```python
from build123d import *

# Parameters (mm, degrees)
CUT_EXTRUDE1_DEPTH      = 7
CUT_EXTRUDE3_DEPTH      = 7
CUT_EXTRUDE3_DEPTH_BACK = 7
SKETCH9_R               = 0.79375


with BuildPart() as part:
    # Sketch2 → Revolve1 (revolve)
    with BuildSketch(Plane(origin=(0, 0, 0), x_dir=(0, 0, -1), z_dir=(1, 0, 0))):
        Polygon((-12, 0), (-12, 6.1), (-11.6, 6.5), (-4.4, 6.5), (-4, 6.1), (-4, 4), (10.75, 4), (12, 2.75), (12, 0), align=None)
    revolve(axis=Axis((0, 0, -12), (0, 0, 1)))

    # Sketch3 → Cut-Extrude1 (cut)
    with BuildSketch(Plane.XY.offset(12)):
        Polygon((3, -1.732050808), (3, 1.732050808), (0, 3.464101615), (-3, 1.732050808), (-3, -1.732050808), (0, -3.464101615), align=None)
    extrude(amount=-CUT_EXTRUDE1_DEPTH, mode=Mode.SUBTRACT)

    # Cut-Extrude2 cone 1 section (through the dimple's axis) → Cut-Extrude2 (revolve, cut)
    with BuildSketch(Plane(origin=(0, 0, 12), x_dir=(0, -1, 0), z_dir=(1, 0, 0))):
        Polygon((0, 0), (3.464101615, 0), (0, 3.464101615), align=None)
    revolve(axis=Axis((0, 0, 12), (0, 0, -1)), mode=Mode.SUBTRACT)

    # Sketch9 → Cut-Extrude3 (cut, two sides: drawn at the far end of the back side and taken through both)
    with BuildSketch(Plane(origin=(0, 0, 0), x_dir=(1, 0, 0), z_dir=(0, 1, 0)).offset(-CUT_EXTRUDE3_DEPTH_BACK)):
        with Locations(Location((0, -8, 0), (0, 0, 90))):
            Circle(SKETCH9_R)
    extrude(amount=CUT_EXTRUDE3_DEPTH + CUT_EXTRUDE3_DEPTH_BACK, mode=Mode.SUBTRACT)


solid = part.part
```
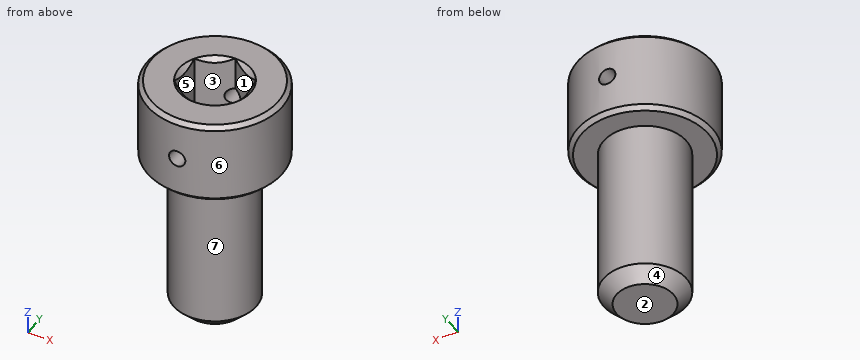
The listing builds one solid part. Answer for the finished solid, in the listing's coordinates (mm). Face numbers are marked on the shaded views. A direction names the side the tool comes from. Coordinates: 2 decimals unless noted, no trailing zeros. Loops run counter-clockwise (first coordinate to the right, second up) from the corner with the lowest first, then second, coordinate; pieces in that order, holes last. Notation, with made-up numbers: (33.5, 14.5) - (79.5, 14.5) arc R16 ccw to (79.5, 32.5) - close; hole circle Ø2 at (30.25, 81.5). An arc over 180 degrees is marked (long way). Write item = value, one per line.
1) Find the intervals of material crossed by line 1 along Y through (x, z) = (1.25, 8.75); line 2 along Z through (x, y) = (-1.75, -5.5); line 3 along X through (y, z) = (1, 11.25), in increasing order.
Responses:
line_1 = -6.38 to -2.74, 2.74 to 6.38
line_2 = 4 to 12
line_3 = -6.42 to -3, 3 to 6.42
2) Section B-B (y = 0) is taken. Determine the outline of the cut face in (x, z).
Responses:
outline = (-6.5, 4.4) - (-6.1, 4) - (-4, 4) - (-4, -10.75) - (-2.75, -12) - (2.75, -12) - (4, -10.75) - (4, 4) - (6.1, 4) - (6.5, 4.4) - (6.5, 11.6) - (6.1, 12) - (3.46, 12) - (3, 11.54) - (3, 5) - (-3, 5) - (-3, 11.54) - (-3.46, 12) - (-6.1, 12) - (-6.5, 11.6) - close
3) Section C-C (z = -8.5) is taken. Determine the outline of the cut face in (x, y), plus the area to 3 significant figures.
Responses:
outline = circle Ø8 at (0, 0)
area = 50.3 mm^2
4) Which of the six approach directions +Z, -Z, +X, -X, +Y, -Y give full straight-line access (tool end or side, diameter ignored) to the marked faces 5, 6 and 7?
Responses:
face_5 = +Z
face_6 = +Z, -Z
face_7 = -Z
5) Each of these flat-tipped pins is pushed along its axis until it touches: P1, Ø3, axis at x = 0.5, y = 0, coming from the +Z side; P2, Ø3, axis at y = 3, z = -7.5, coming from the -X side; P3, Ø3, axis at x = -1, z = -4, coming from the +Y side. Where does it stop, or does it pass through?
Responses:
P1 = 5
P2 = -3.71
P3 = 4
6) Determine the mould class of the marked faces 1, 2, 3 and 4 for opening direction X: pulls with the +X half, pulls with the -X half, needs draft (parallel to the pull), parting line crosses it, or undercut.
Responses:
face_1 = undercut
face_2 = needs draft
face_3 = undercut
face_4 = parting line crosses it
7) Section A-A (z = 8) is taken. Determine the outline of the cut face in (x, y), plus the area to 3 significant figures.
Responses:
outline = (-3, -1.73) - (-3, 1.73) - (-0.79, 3.01) - (-0.79, 6.45) arc R6.5 ccw to (-0.79, -6.45) - (-0.79, -3.01) - close; (0.79, -6.45) arc R6.5 ccw to (0.79, 6.45) - (0.79, 3.01) - (3, 1.73) - (3, -1.73) - (0.79, -3.01) - close
area = 91.2 mm^2
